CAD build for the part. Positions are in the model's coordinates, mm. A direction names the side the tool comes from. Give positions to 0.01 mm unless a question says otherwise; leave off trailing zeros. Answer as CSV lines item,"result".
```python
from build123d import *

# Parameters (mm, degrees)
SKETCH1_R           = 63.001442855
BOSS_EXTRUDE1_DEPTH = 10
BOSS_EXTRUDE2_DEPTH = 7
BOSS_EXTRUDE3_DEPTH = 5


with BuildPart() as part:
    # Sketch1 → Boss-Extrude1 (new body)
    with BuildSketch(Plane.XY):
        Circle(SKETCH1_R)
    extrude(amount=BOSS_EXTRUDE1_DEPTH)

    # Sketch1_3 → Boss-Extrude2 (add)
    with BuildSketch(Plane.XY):
        with BuildLine():
            ThreePointArc((-51.791249261, -35.872667893), (-63.001442855, 0), (-51.791249261, 35.872667893))
            add(Edge.make_bspline(
                [(-51.791249261, 35.872667893), (-69.091772014, 50.033080135), (-85.201999092, 48.884507071), (-100.829128316, 41.764792431)],
                knots=[0, 0, 0, 0, 0.38504414, 0.38504414, 0.38504414, 0.38504414], degree=3))
            add(Edge.make_bspline(
                [(-100.829128316, 41.764792431), (-125.787292045, 30.393861714), (-149.513196882, 3.792078212), (-174.887829117, 0)],
                knots=[0.38504414, 0.38504414, 0.38504414, 0.38504414, 1, 1, 1, 1], degree=3))
            add(Edge.make_bspline(
                [(-100.829128316, -41.764792431), (-125.787292045, -30.393861714), (-149.513196882, -3.792078212), (-174.887829117, 0)],
                knots=[0.38504414, 0.38504414, 0.38504414, 0.38504414, 1, 1, 1, 1], degree=3))
            add(Edge.make_bspline(
                [(-51.791249261, -35.872667893), (-69.091772014, -50.033080135), (-85.201999092, -48.884507071), (-100.829128316, -41.764792431)],
                knots=[0, 0, 0, 0, 0.38504414, 0.38504414, 0.38504414, 0.38504414], degree=3))
        make_face()
        with BuildLine():
            ThreePointArc((-35.872667893, 51.791249261), (0, 63.001442855), (35.872667893, 51.791249261))
            add(Edge.make_bspline(
                [(35.872667893, 51.791249261), (50.033080135, 69.091772014), (48.884507071, 85.201999092), (41.764792431, 100.829128316)],
                knots=[0, 0, 0, 0, 0.38504414, 0.38504414, 0.38504414, 0.38504414], degree=3))
            add(Edge.make_bspline(
                [(41.764792431, 100.829128316), (30.393861714, 125.787292045), (3.792078212, 149.513196882), (0, 174.887829117)],
                knots=[0.38504414, 0.38504414, 0.38504414, 0.38504414, 1, 1, 1, 1], degree=3))
            add(Edge.make_bspline(
                [(-41.764792431, 100.829128316), (-30.393861714, 125.787292045), (-3.792078212, 149.513196882), (0, 174.887829117)],
                knots=[0.38504414, 0.38504414, 0.38504414, 0.38504414, 1, 1, 1, 1], degree=3))
            add(Edge.make_bspline(
                [(-35.872667893, 51.791249261), (-50.033080135, 69.091772014), (-48.884507071, 85.201999092), (-41.764792431, 100.829128316)],
                knots=[0, 0, 0, 0, 0.38504414, 0.38504414, 0.38504414, 0.38504414], degree=3))
        make_face()
        with BuildLine():
            ThreePointArc((51.791249261, 35.872667893), (60.133623009, 18.79173184), (63.001442855, 0))
            ThreePointArc((63.001442855, 0), (60.133623009, -18.79173184), (51.791249261, -35.872667893))
            add(Edge.make_bspline(
                [(51.791249261, -35.872667893), (69.091772014, -50.033080135), (85.201999092, -48.884507071), (100.829128316, -41.764792431)],
                knots=[0, 0, 0, 0, 0.38504414, 0.38504414, 0.38504414, 0.38504414], degree=3))
            add(Edge.make_bspline(
                [(100.829128316, -41.764792431), (125.787292045, -30.393861714), (149.513196882, -3.792078212), (174.887829117, 0)],
                knots=[0.38504414, 0.38504414, 0.38504414, 0.38504414, 1, 1, 1, 1], degree=3))
            add(Edge.make_bspline(
                [(100.829128316, 41.764792431), (125.787292045, 30.393861714), (149.513196882, 3.792078212), (174.887829117, 0)],
                knots=[0.38504414, 0.38504414, 0.38504414, 0.38504414, 1, 1, 1, 1], degree=3))
            add(Edge.make_bspline(
                [(51.791249261, 35.872667893), (69.091772014, 50.033080135), (85.201999092, 48.884507071), (100.829128316, 41.764792431)],
                knots=[0, 0, 0, 0, 0.38504414, 0.38504414, 0.38504414, 0.38504414], degree=3))
        make_face()
        with BuildLine():
            add(Edge.make_bspline(
                [(35.872667893, -51.791249261), (50.033080135, -69.091772014), (48.884507071, -85.201999092), (41.764792431, -100.829128316)],
                knots=[0, 0, 0, 0, 0.38504414, 0.38504414, 0.38504414, 0.38504414], degree=3))
            ThreePointArc((35.872667893, -51.791249261), (0, -63.001442855), (-35.872667893, -51.791249261))
            add(Edge.make_bspline(
                [(-35.872667893, -51.791249261), (-50.033080135, -69.091772014), (-48.884507071, -85.201999092), (-41.764792431, -100.829128316)],
                knots=[0, 0, 0, 0, 0.38504414, 0.38504414, 0.38504414, 0.38504414], degree=3))
            add(Edge.make_bspline(
                [(-41.764792431, -100.829128316), (-30.393861714, -125.787292045), (-3.792078212, -149.513196882), (0, -174.887829117)],
                knots=[0.38504414, 0.38504414, 0.38504414, 0.38504414, 1, 1, 1, 1], degree=3))
            add(Edge.make_bspline(
                [(41.764792431, -100.829128316), (30.393861714, -125.787292045), (3.792078212, -149.513196882), (0, -174.887829117)],
                knots=[0.38504414, 0.38504414, 0.38504414, 0.38504414, 1, 1, 1, 1], degree=3))
        make_face()
    extrude(amount=BOSS_EXTRUDE2_DEPTH)

    # Sketch1_4 → Boss-Extrude3 (add)
    with BuildSketch(Plane.XY):
        with BuildLine():
            ThreePointArc((-51.791249261, 35.872667893), (-44.548747467, 44.548747467), (-35.872667893, 51.791249261))
            add(Edge.make_bspline(
                [(-35.872667893, 51.791249261), (-50.033080135, 69.091772014), (-48.884507071, 85.201999092), (-41.764792431, 100.829128316)],
                knots=[0, 0, 0, 0, 0.38504414, 0.38504414, 0.38504414, 0.38504414], degree=3))
            add(Edge.make_bspline(
                [(-41.764792431, 100.829128316), (-67.453341468, 110.436752916), (-103.040391174, 108.403199611), (-123.664369915, 123.664369915)],
                knots=[0.38504414, 0.38504414, 0.38504414, 0.38504414, 1, 1, 1, 1], degree=3))
            add(Edge.make_bspline(
                [(-100.829128316, 41.764792431), (-110.436752916, 67.453341468), (-108.403199611, 103.040391174), (-123.664369915, 123.664369915)],
                knots=[0.38504414, 0.38504414, 0.38504414, 0.38504414, 1, 1, 1, 1], degree=3))
            add(Edge.make_bspline(
                [(-51.791249261, 35.872667893), (-69.091772014, 50.033080135), (-85.201999092, 48.884507071), (-100.829128316, 41.764792431)],
                knots=[0, 0, 0, 0, 0.38504414, 0.38504414, 0.38504414, 0.38504414], degree=3))
        make_face()
        with BuildLine():
            ThreePointArc((35.872667893, 51.791249261), (44.548747467, 44.548747467), (51.791249261, 35.872667893))
            add(Edge.make_bspline(
                [(51.791249261, 35.872667893), (69.091772014, 50.033080135), (85.201999092, 48.884507071), (100.829128316, 41.764792431)],
                knots=[0, 0, 0, 0, 0.38504414, 0.38504414, 0.38504414, 0.38504414], degree=3))
            add(Edge.make_bspline(
                [(100.829128316, 41.764792431), (110.436752916, 67.453341468), (108.403199611, 103.040391174), (123.664369915, 123.664369915)],
                knots=[0.38504414, 0.38504414, 0.38504414, 0.38504414, 1, 1, 1, 1], degree=3))
            add(Edge.make_bspline(
                [(41.764792431, 100.829128316), (67.453341468, 110.436752916), (103.040391174, 108.403199611), (123.664369915, 123.664369915)],
                knots=[0.38504414, 0.38504414, 0.38504414, 0.38504414, 1, 1, 1, 1], degree=3))
            add(Edge.make_bspline(
                [(35.872667893, 51.791249261), (50.033080135, 69.091772014), (48.884507071, 85.201999092), (41.764792431, 100.829128316)],
                knots=[0, 0, 0, 0, 0.38504414, 0.38504414, 0.38504414, 0.38504414], degree=3))
        make_face()
        with BuildLine():
            add(Edge.make_bspline(
                [(51.791249261, -35.872667893), (69.091772014, -50.033080135), (85.201999092, -48.884507071), (100.829128316, -41.764792431)],
                knots=[0, 0, 0, 0, 0.38504414, 0.38504414, 0.38504414, 0.38504414], degree=3))
            ThreePointArc((51.791249261, -35.872667893), (44.548747467, -44.548747467), (35.872667893, -51.791249261))
            add(Edge.make_bspline(
                [(35.872667893, -51.791249261), (50.033080135, -69.091772014), (48.884507071, -85.201999092), (41.764792431, -100.829128316)],
                knots=[0, 0, 0, 0, 0.38504414, 0.38504414, 0.38504414, 0.38504414], degree=3))
            add(Edge.make_bspline(
                [(41.764792431, -100.829128316), (67.453341468, -110.436752916), (103.040391174, -108.403199611), (123.664369915, -123.664369915)],
                knots=[0.38504414, 0.38504414, 0.38504414, 0.38504414, 1, 1, 1, 1], degree=3))
            add(Edge.make_bspline(
                [(100.829128316, -41.764792431), (110.436752916, -67.453341468), (108.403199611, -103.040391174), (123.664369915, -123.664369915)],
                knots=[0.38504414, 0.38504414, 0.38504414, 0.38504414, 1, 1, 1, 1], degree=3))
        make_face()
        with BuildLine():
            add(Edge.make_bspline(
                [(-35.872667893, -51.791249261), (-50.033080135, -69.091772014), (-48.884507071, -85.201999092), (-41.764792431, -100.829128316)],
                knots=[0, 0, 0, 0, 0.38504414, 0.38504414, 0.38504414, 0.38504414], degree=3))
            ThreePointArc((-35.872667893, -51.791249261), (-44.548747467, -44.548747467), (-51.791249261, -35.872667893))
            add(Edge.make_bspline(
                [(-51.791249261, -35.872667893), (-69.091772014, -50.033080135), (-85.201999092, -48.884507071), (-100.829128316, -41.764792431)],
                knots=[0, 0, 0, 0, 0.38504414, 0.38504414, 0.38504414, 0.38504414], degree=3))
            add(Edge.make_bspline(
                [(-100.829128316, -41.764792431), (-110.436752916, -67.453341468), (-108.403199611, -103.040391174), (-123.664369915, -123.664369915)],
                knots=[0.38504414, 0.38504414, 0.38504414, 0.38504414, 1, 1, 1, 1], degree=3))
            add(Edge.make_bspline(
                [(-41.764792431, -100.829128316), (-67.453341468, -110.436752916), (-103.040391174, -108.403199611), (-123.664369915, -123.664369915)],
                knots=[0.38504414, 0.38504414, 0.38504414, 0.38504414, 1, 1, 1, 1], degree=3))
        make_face()
    extrude(amount=BOSS_EXTRUDE3_DEPTH)


solid = part.part
```
1) Pin check, flat tips, straight feed: P1, Ø3, axis at y = -67, z = 3, coming from the +X side; P2, Ø5, axis at x = 102, z = 8.5, coming from the +Y side; P3, Ø3, axis at x = 80, z = 2, coming from the -Y side. Stop position of each tip, or through.
Data:
P1,"stops at x = 107.4"
P2,"stops at y = 42.14"
P3,"stops at y = -109.59"
2) Wall check: line 1 along X through (y, z) = (-1, 8.5); line 2 along Z through (x, y) = (16.5, -102.5); line 3 along Z through (x, y) = (46.5, 50). Give the ranges that are in metal, low to high. Write a range as [from, to].
Data:
line 1,"x = [-62.99, 62.99]"
line 2,"z = [0, 7]"
line 3,"z = [0, 5]"
3) Which spindle directions (+Z, -Z, +X, -X, +Y, -Y) get a long thin tool onto all of the face, cutting with end or side? Do faces 1 (the cylindrical face through (-62.94, 2.77, 8.02)), 2 (the flat face through (-1, 1, 10)). Say none if no direction does.
Data:
face 1,"+Z"
face 2,"+Z, +X, -X, +Y, -Y"
